```python
from build123d import *

# Parameters (mm, degrees)
ESTRUSIONE_ESTRUSIONE2_DEPTH = 1.5


with BuildPart() as part:
    # Schizzo3 → Estrusione-Estrusione2 (new body, symmetric)
    with BuildSketch(Plane(origin=(0, 0, 0), x_dir=(1, 0, 0), z_dir=(0, 1, 0))):
        Polygon((-20, -3.5), (-20, -6.5), (-12, -6.5), (-12, -3.5), (-4, -3.5), (-4, -6.5), (4, -6.5), (4, -3.5), (12, -3.5), (12, -6.5), (20, -6.5), (20, -3.5), (20, 3.5), (20, 6.5), (12, 6.5), (12, 3.5), (4, 3.5), (4, 6.5), (-4, 6.5), (-4, 3.5), (-12, 3.5), (-12, 6.5), (-20, 6.5), (-20, 3.5), align=None)
    extrude(amount=ESTRUSIONE_ESTRUSIONE2_DEPTH, both=True)


solid = part.part
```
Work out the finished part from the listing and answer in its coordinate system (mm). A direction names the side the tool comes from. Give positions to 0.01 mm unless a question says otherwise; leave off trailing zeros. Order: outer loops, then holes, each group sorted by start corner. A loop starts at its lowest first (then second) coordinate and runs counter-clockwise, first axis right, second up. Notation, with made-up numbers: (70.5, -2.75) - (96.5, -2.75) arc R20 ccw to (96.5, 21.25) - close; hole circle Ø3 at (-14.5, 86.5). An arc over 180 degrees is marked (long way). One line per item, written item: value. Start each with the question number.
1. Each of these flat-tipped pins is pushed along its axis until it touches: pin 1 Ø0.9 at (x, y) = (8.5, 0.5) entering from +Z; pin 2 Ø1.5 at (x, y) = (6.5, -0.5) entering from -Z. Where does it stop, or does it pass through?
2. Which of the six approach directions +Z, -Z, +X, -X, +Y, -Y give full straight-line access (tool end or side, diameter ignored) to faces 4 (the face through (0, 0, -6.5)), 5 (the face through (-4, 0, 5)), 6 (the face through (-8, 0, -3.5))?
3. Consider line 1 (X direction, y = 0.7, z = 5.75); line 2 (Z direction, x = -10.5, y = -1.3). Determine where each line is inside the solid, lowest interval first.
4. Section B-B, the plane x = -6.5 is taken. Write down the section's boundary in (y, z), then the cut area to 3 significant figures.
5. Section A-A, the plane z = -4.5 is taken. Write down the section's boundary in (x, y), then the cut area to 3 significant figures.
6. For a pull along X with two mould halves and no side action, classify faces 1 (the face through (-16, 0, 6.5)), 2 (the face through (-20, 0, 0)), 3 (the face through (12, 0, -5)) as released by +X, released by -X, zero draft, split by the parting line, or undercut.
Filled sheet:
1. pin 1: z = 3.5
1. pin 2: z = -3.5
2. face 4: -Z, +X, -X, +Y, -Y
2. face 5: +Z, +Y, -Y
2. face 6: -Z, +Y, -Y
3. line 1: -20 to -12, -4 to 4, 12 to 20
3. line 2: -3.5 to 3.5
4. outline: (-1.5, -3.5) - (1.5, -3.5) - (1.5, 3.5) - (-1.5, 3.5) - close
4. area: 21.0 mm²
5. outline: (-20, -1.5) - (-12, -1.5) - (-12, 1.5) - (-20, 1.5) - close; (-4, -1.5) - (4, -1.5) - (4, 1.5) - (-4, 1.5) - close; (12, -1.5) - (20, -1.5) - (20, 1.5) - (12, 1.5) - close
5. area: 72.0 mm²
6. face 1: zero draft
6. face 2: released by -X
6. face 3: undercut
